Geometry: final body of the model. Coordinates: model frame, mm. Give positions to 0.01 mm unless a question says otherwise; leave off trailing zeros. Write each loop counter-clockwise with the first axis right and the second up, starting at its lowest first coordinate (ties: lowest second). Pieces come first, ordered by that corner, then holes. Notation, with made-up numbers: M -9,22.5 L 2,22.5 A15 ccw 2,27.5 Z; hole C 89,42 d9. An arc over 180 degrees is marked long. One line per question, with ' | ' between items.
from build123d import *

# Parameters (mm, degrees)
CYLINDER019_W               = 10
CYLINDER019_H               = 10
CYLINDER019_ANGLE           = 120
CYLINDER019_PLACEMENT_ANGLE = 30
CYLINDER017_W               = 12
CYLINDER017_H               = 10
CYLINDER017_ANGLE           = 120
CYLINDER017_PLACEMENT_ANGLE = 30


with BuildPart() as cilindro010:
    # Cylinder019 → Cylinder019 (revolve)
    with BuildSketch(Plane.XZ):
        with Locations((5, 5)):
            Rectangle(CYLINDER019_W, CYLINDER019_H)
    revolve(axis=Axis((0, 0, 0), (0, 0, 1)), revolution_arc=CYLINDER019_ANGLE)


with BuildPart() as cilindro010_1:
    # Cylinder019 placement: moved
    add(cilindro010.part.moved(Location((-30.75, -30, 0))).rotate(Axis((-30.75, -30, 0), (0, 0, 1)), CYLINDER019_PLACEMENT_ANGLE))


with BuildPart() as obj1:
    # Cylinder017 → Cylinder017 (revolve)
    with BuildSketch(Plane.XZ):
        with Locations((6, 5)):
            Rectangle(CYLINDER017_W, CYLINDER017_H)
    revolve(axis=Axis((0, 0, 0), (0, 0, 1)), revolution_arc=CYLINDER017_ANGLE)


with BuildPart() as obj1_1:
    # Cylinder017 placement: moved
    add(obj1.part.moved(Location((-30.75, -30, 0))).rotate(Axis((-30.75, -30, 0), (0, 0, 1)), CYLINDER017_PLACEMENT_ANGLE))

    # Cut006: cut Cilindro010
    add(cilindro010_1.part, mode=Mode.SUBTRACT)


solid = obj1_1.part
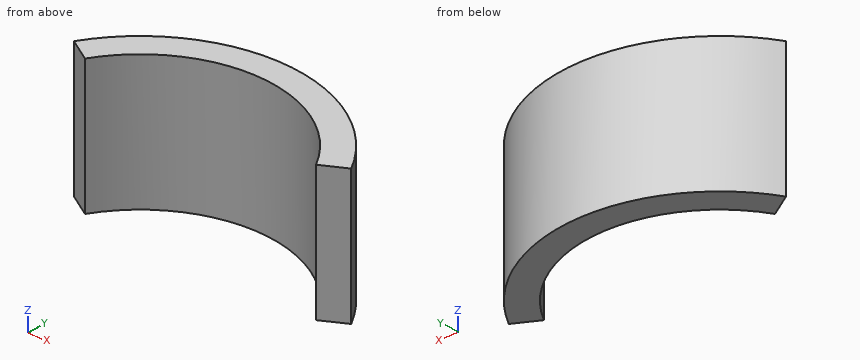
(1) Cut plane A-A, the plane y = -22.75. Return loops of the section in (x, z).
Working result:
outline: M -40.31,0 L -37.64,0 L -37.64,10 L -40.31,10 Z; M -23.86,0 L -21.19,0 L -21.19,10 L -23.86,10 Z
(2) Material intervals for L1, parallel to X at y = -21.5, z = 1.25; L2, parallel to X at y = -23.5, z = 1.25; L3, parallel to Y at x = -30.5, z = 3, sorted ascending. Write a range as [from, to].
Working result:
L1: x = [-39.22, -36.02], [-25.48, -22.28] | L2: x = [-40.84, -38.35], [-23.15, -20.66] | L3: y = [-20, -18]
(3) Cut plane D-D, the plane x = -22.5. Return loops of the section in (y, z), then the cut area to 3 significant figures.
Working result:
outline: M -24.35,0 L -21.29,0 L -21.29,10 L -24.35,10 Z | area: 30.6 mm^2
(4) Cut plane C-C, the plane y = -21. Return loops of the section in (x, z), then the cut area to 3 significant figures.
Working result:
outline: M -38.69,0 L -35.11,0 L -35.11,10 L -38.69,10 Z; M -26.39,0 L -22.81,0 L -22.81,10 L -26.39,10 Z | area: 71.6 mm^2
(5) Cut plane B-B, the plane z = 4.5. Return loops of the section in (x, y), then the cut area to 3 significant figures.
Working result:
outline: M -41.14,-24 L -39.41,-25 A10 cw -22.09,-25 L -20.36,-24 A12 ccw Z | area: 46.1 mm^2
(6) First-contact query: P1, Ø1, axis at y = -22.5, z = 7.5, coming from the -X side; P2, Ø3, axis at y = -24, z = 3, coming from the -X side. Flat tips, straight axial feed; report the tip coordinate or a pass-through.
Working result:
P1: stops at x = -40.5 | P2: stops at x = -41.14
